Work out the finished part from the listing and answer in its coordinate system (mm). Face numbers are marked on the shaded views. A direction names the side the tool comes from. Round coordinates to 2 decimals unless told otherwise and drop trailing zeros. Order: outer loops, then holes, each group sorted by start corner. A loop starts at its lowest first (then second) coordinate and runs counter-clockwise, first axis right, second up. Notation, with made-up numbers: (40, 14.25) - (75, 14.25) arc R16 ccw to (75, 24.25) - close; hole circle Ø7 at (10, 64.25). An arc over 180 degrees is marked (long way). Put each result on its own line as item: value.
```python
from build123d import *

# Parameters (mm, degrees)
F1_R     = 1.825
F1_W     = 5.875
F1_H     = 5.75
F2_DEPTH = 9.75
F3_DEPTH = 2.25
F4_R     = 2.975
F4_R_2   = 1.825
F5_DEPTH = 3


with BuildPart() as f2:
    # F1 (on Top) → F2 (new body)
    with BuildSketch(Plane.XY):
        Polygon((-7.875, 3.0625), (-7.875, 5.9375), (-16.075, 5.9375), (-16.075, -5.9375), (-7.875, -5.9375), (-7.875, -2.6875), (-5.875, -2.6875), (-5.875, 3.0625), align=None)
        with Locations((-12.125, 0)):
            Circle(F1_R, mode=Mode.SUBTRACT)
        with Locations((-2.9375, 0.1875)):
            Rectangle(F1_W, F1_H)
        Polygon((-7.875, -5.9375), (0, -5.9375), (0, -2.6875), (-5.875, -2.6875), (-7.875, -2.6875), align=None)
        Polygon((0, -5.9375), (7.875, -5.9375), (7.875, -2.6875), (5.875, -2.6875), (0, -2.6875), align=None)
        Polygon((0, 3.0625), (0, 5.9375), (-7.875, 5.9375), (-7.875, 3.0625), (-5.875, 3.0625), align=None)
        Polygon((7.875, 3.0625), (7.875, 5.9375), (0, 5.9375), (0, 3.0625), (5.875, 3.0625), align=None)
        with Locations((2.9375, 0.1875)):
            Rectangle(F1_W, F1_H)
        Polygon((16.075, -5.9375), (16.075, 5.9375), (7.875, 5.9375), (7.875, 3.0625), (5.875, 3.0625), (5.875, -2.6875), (7.875, -2.6875), (7.875, -5.9375), align=None)
        with Locations((12.125, 0)):
            Circle(F1_R, mode=Mode.SUBTRACT)
    extrude(amount=-F2_DEPTH)

    # F1 (on Top) → F3 (join)
    with BuildSketch(Plane.XY):
        with Locations((-2.9375, 0.1875)):
            Rectangle(F1_W, F1_H)
        with Locations((2.9375, 0.1875)):
            Rectangle(F1_W, F1_H)
    extrude(amount=F3_DEPTH)

    # F4 (on face) → F5 (cut)
    with BuildSketch(Plane(origin=(0, 0, -9.75), x_dir=(1, 0, 0), z_dir=(0, 0, -1))):
        with Locations((12.125, 0)):
            Circle(F4_R)
        with Locations((12.125, 0)):
            Circle(F4_R_2, mode=Mode.SUBTRACT)
        with Locations((-12.125, 0)):
            Circle(F4_R)
        with Locations((-12.125, 0)):
            Circle(F4_R_2, mode=Mode.SUBTRACT)
        with Locations((12.125, 0)):
            Circle(F4_R_2)
        with Locations((-12.125, 0)):
            Circle(F4_R_2)
    extrude(amount=-F5_DEPTH, mode=Mode.SUBTRACT)


solid = f2.part
```
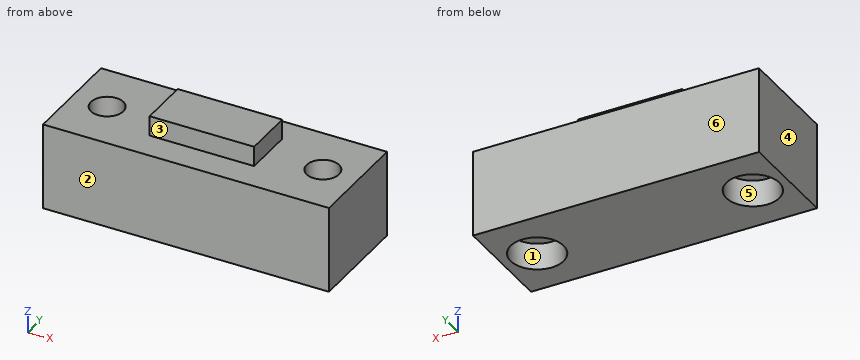
1) A cutting plane is placed at B-B on x = 13. Write down the section's boundary in (y, z).
Findings below:
outline: (-5.94, -9.75) - (-2.84, -9.75) - (-2.84, -6.75) - (-1.6, -6.75) - (-1.6, 0) - (-5.94, 0) - close; (1.6, -6.75) - (2.84, -6.75) - (2.84, -9.75) - (5.94, -9.75) - (5.94, 0) - (1.6, 0) - close
2) For the marked faces 1, 2 and 3, determine the directions among +Z, -Z, +X, -X, +Y, -Y from which every point of the face is accessible in a straight line to the end or side of a thin tool.
Findings below:
face 1: -Z
face 2: +Z, -Z, +X, -X, -Y
face 3: +Z, +X, -X, -Y
3) A cutting plane is placed at C-C on z = -3. Give the number of separate pieces and of enclosed holes in the cut face, then the cut area to 3 significant figures.
Findings below:
separate pieces: 1
enclosed holes: 2
area: 361 mm2
4) For a pull along Y with two mould halves and no side action, classify the marked faces 4, 5 and 6 as pulls with the +Y half, pulls with the -Y half, needs draft (parallel to the pull), parting line crosses it, or undercut.
Findings below:
face 4: needs draft
face 5: undercut
face 6: pulls with the +Y half
5) A cutting plane is placed at D-D on x = 2. Write down the section's boundary in (y, z).
Findings below:
outline: (-5.94, -9.75) - (5.94, -9.75) - (5.94, 0) - (3.06, 0) - (3.06, 2.25) - (-2.69, 2.25) - (-2.69, 0) - (-5.94, 0) - close
6) Given pin 1 Ø1.8 at (y, z) = (-1, 1) entering from +X (3 decimals); pin 2 Ø4 at (x, y) = (-12.125, 0) entering from +Z; pin 3 Ø1.1 at (y, z) = (-1, 1) entering from -X (3 decimals), each flat-ended and moving along its own axis, determine where each tip first touches the part or whether it passes through.
Findings below:
pin 1: stops at x = 5.875
pin 2: stops at z = 0
pin 3: stops at x = -5.875
7) Straight lines are drawn through the part: L1, parallel to X at y = 0, z = -7.6 (3 decimals); L2, parallel to Z at x = 6, y = 3.75; L3, parallel to X at y = 1.25, z = -6 (3 decimals). For each, find the intervals that lie inside material, in ascending order. Write a range as from..to.
Findings below:
L1: x = -16.075..-15.1, -9.15..9.15, 15.1..16.075
L2: z = -9.75..0
L3: x = -16.075..-13.455, -10.795..10.795, 13.455..16.075
8) A cutting plane is placed at A-A on y = 0. Write down the section's boundary in (x, z) (3 decimals).
Findings below:
outline: (-16.075, -9.75) - (-15.1, -9.75) - (-15.1, -6.75) - (-13.95, -6.75) - (-13.95, 0) - (-16.075, 0) - close; (-10.3, -6.75) - (-9.15, -6.75) - (-9.15, -9.75) - (9.15, -9.75) - (9.15, -6.75) - (10.3, -6.75) - (10.3, 0) - (5.875, 0) - (5.875, 2.25) - (-5.875, 2.25) - (-5.875, 0) - (-10.3, 0) - close; (13.95, -6.75) - (15.1, -6.75) - (15.1, -9.75) - (16.075, -9.75) - (16.075, 0) - (13.95, 0) - close
